Geometry: final body of the model. Coordinates: model frame, mm. Round coordinates to 2 decimals unless told otherwise and drop trailing zeros. Write each loop counter-clockwise with the first axis right and the second up, starting at its lowest first coordinate (ties: lowest second). Pieces come first, ordered by that corner, then holes. Notation, with made-up numbers: M -29.5,13 L 20.5,13 A24 cw 20.5,37 Z; hole C 12.5,-36.5 d9. An arc over 180 degrees is marked long. Put each result on its own line as item: value. Start each with the question number.
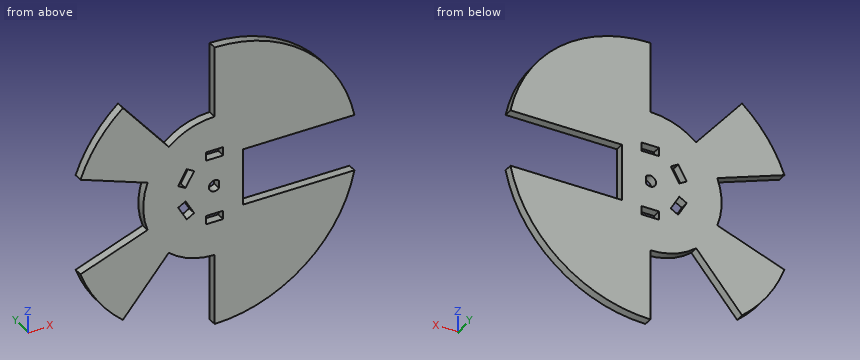
Autodesk Inventor part; units mm, degrees
ref_plane "YZ Plane" through (0, 0, 0) normal (1, 0, 0) x (0, 1, 0)
ref_plane "XZ Plane" through (0, 0, 0) normal (0, 1, 0) x (-1, 0, 0)
ref_plane "XY Plane" through (0, 0, 0) normal (0, 0, 1) x (1, 0, 0)
sketch "草圖1" plane through (0, 0, 0) normal (0, 1, 0) x (-1, 0, 0)
  circle A0 centre (0, 0) radius 50
  circle A1 centre (0, 0) radius 25
  line L0 (-50, 10) -> (-10, 10)
  line L1 (-10, 10) -> (-10, -10)
  line L2 (-10, -10) -> (-50, -10)
  line L3 (-50, -10) -> (-50, 10)
  line L4 (0, 0) -> (0, -50)
  line L5 (0, 0) -> (32.1394, -38.3022)
  arc A2 (0, -50) -> (32.1394, -38.3022) centre (0, 0) ccw
  line L6 (0, 0) -> (46.9846, -17.101)
  line L7 (0, 0) -> (46.9846, 17.101)
  arc A3 (46.9846, -17.101) -> (46.9846, 17.101) centre (0, 0) ccw
  line L8 (0, 0) -> (32.1394, 38.3022)
  line L9 (0, 0) -> (0, 50)
  arc A4 (32.1394, 38.3022) -> (0, 50) centre (0, 0) ccw
  circle A5 centre (0, 0) radius 2
  line L10 (-1.5, 1.3229) -> (-1.5, -1.3229)
  point P0 (16.0697, -19.1511)
  point P1 (0, -25)
  point P2 (-48.9898, 10)
  point P3 (-48.9898, -10)
  point P4 (16.0697, 19.1511)
  point P5 (0, 25)
  point P6 (23.4923, -8.5505)
  point P7 (23.4923, 8.5505)
  point P8 (-50, 0)
  dimension "d0" = 100
  dimension "d1" = 50
  dimension "d2" = 20
  dimension "d3" = 40
  dimension "d5" = 40
  dimension "d6" = 50
  dimension "d9" = 140
  dimension "d28" = 4
  dimension "d29" = 1.5
  dimension "d30" = 50
extrude "擠出1" add sketch "草圖1" along normal blind 3 contours L7 A1 L8 A0 | A0 L5 A1 L6 | L7 A5 L8 A1 | A1 L6 A5 L7 | A1 L5 A5 L6 | L9 A1 L0 A0 | L8 A5 L9 A1 | A0 L2 A1 L4 | A1 L4 A5 L5 | L9 A5 L4 A1 L2 L1 L0 | L10 A5
sketch "草圖2" plane through (0, 3, 0) normal (0, 1, 0) x (1, 0, 0)
  line L0 (-3, 13) -> (3, 13)
  line L1 (3, 13) -> (3, 10)
  line L2 (3, 10) -> (-3, 10)
  line L3 (-3, 10) -> (-3, 13)
  line L4 (-12.7583, 3.9019) -> (-9.7583, 9.0981)
  line L5 (-9.7583, 9.0981) -> (-7.1603, 7.5981)
  line L6 (-7.1603, 7.5981) -> (-10.1603, 2.4019)
  line L7 (-10.1603, 2.4019) -> (-12.7583, 3.9019)
  line L8 (-9.7583, -9.0981) -> (-12.7583, -3.9019)
  line L9 (-12.7583, -3.9019) -> (-10.1603, -2.4019)
  line L10 (-10.1603, -2.4019) -> (-7.1603, -7.5981)
  line L11 (-7.1603, -7.5981) -> (-9.7583, -9.0981)
  line L12 (3, -13) -> (-3, -13)
  line L13 (-3, -13) -> (-3, -10)
  line L14 (-3, -10) -> (3, -10)
  line L15 (3, -10) -> (3, -13)
  point P0 (0, 0)
  point P1 (0, 10)
  point P2 (-8.6603, 5)
  point P3 (-8.6603, -5)
  point P4 (0, -10)
  dimension "d31" = 3
  dimension "d32" = 6
  dimension "d33" = 10
  dimension "d36" = 180
extrude "擠出2" cut sketch "草圖2" against normal through all
properties part number "rolling_plate_small"
1) First-contact query: pin 1 (6 mm diameter, centred on x = -35, z = 12.5, fed in from +Y); pin 2 (0.9 mm diameter, centred on x = -1, y = 1.5, fed in from -Z); pin 3 (1.5 mm diameter, centred on x = 32, y = 1.5, fed in from +Z); pin 4 (0.8 mm diameter, centred on y = 1, z = -0.5, fed in from -X). Flat tips, straight axial feed; report the tip coordinate or a pass-through.
2) Ray query, probe 1 along X at (y, z) = (1.9, 0); probe 2 along X at (y, z) = (2.7, 30.5); probe 3 along Z at (x, y) = (24.5, 0.1). Return the intervals inside material, ascending.
3) Section B-B, the plane z = 0. Output: boundary loops of the cut face in (x, y).
4) Section C-C, the plane y = 1.3. Give the number of separate pieces and of enclosed holes in the cut face, and give its area (3 significant figures).
5) Section A-A, the plane x = 21. Output: boundary loops of the cut face in (y, z), and give its area (3 significant figures).
Solved:
1. pin 1: stops at y = 3
1. pin 2: stops at z = -24.99
1. pin 3: stops at z = 39.03
1. pin 4: stops at x = -25
2. probe 1: x = -25 to -2, 1.5 to 10
2. probe 2: x = -39.62 to -25.59, 0 to 39.62
2. probe 3: z = -43.59 to -10, 10 to 43.59
3. outline: M -25,0 L -2,0 L -2,3 L -25,3 Z; M 1.5,0 L 10,0 L 10,3 L 1.5,3 Z
4. separate pieces: 1
4. enclosed holes: 5
4. area: 5,010 mm2
5. outline: M 0,-45.38 L 3,-45.38 L 3,-10 L 0,-10 Z; M 0,10 L 3,10 L 3,45.38 L 0,45.38 Z
5. area: 212 mm2
